The listing builds one solid part. Answer for the finished solid, in the listing's coordinates (mm). Round coordinates to 2 decimals unless told otherwise and drop trailing zeros. Loops run counter-clockwise (first coordinate to the right, second up) from the corner with the lowest first, then second, coordinate; pieces in that order, holes last. Notation, with made-up numbers: (-27, 35.25) -> (12, 35.25) arc R12 cw to (12, 44.25) -> close; hole circle Ø1 at (-6, 74). An arc over 180 degrees is marked (long way). Write each question's results on one line, items separated by ' | '. Start each with the question number.
(1) Straight lines are drawn through the part: probe 1 along X at (y, z) = (0.25, 183); probe 2 along Y at (x, z) = (-0.5, 208); probe 3 along Y at (x, z) = (-3.25, 251). For each, find the intervals that lie inside material, in ascending order.
(2) Flat-ended cylindrical pins translate along their axes: pin 1 (1.5 mm diameter, centred on y = -1.5, z = 77, fed in from +X); pin 2 (1.5 mm diameter, centred on y = 3.5, z = 240, fed in from +X); pin 3 (6 mm diameter, centred on x = 3.5, z = 210, fed in from +Y). Find the tip coordinate at first contact, or state that the pin passes through.
(3) The part is cut by section A-A (z = 55). Determine the outline of the cut face in (x, y).
```python
from build123d import *

# Parameters (mm, degrees)
CROQUIS1_R              = 5
SALIENTE_EXTRUIR1_DEPTH = 270


with BuildPart() as part:
    # Croquis1 → Saliente-Extruir1 (new body)
    with BuildSketch(Plane.XY):
        Circle(CROQUIS1_R)
    extrude(amount=SALIENTE_EXTRUIR1_DEPTH)

    # Cortar-Barrer1: sweep along a curve in space
    with BuildLine() as cortar_barrer1_path:
        ThreePointArc((5, 0, 270), (3.535533906, 3.535533906, 270), (0, 5, 270))
        ThreePointArc((0, 5, 270), (-3.535533906, 3.535533906, 270), (-5, 0, 270))
        ThreePointArc((-5, 0, 270), (-3.535533906, -3.535533906, 270), (0, -5, 270))
        ThreePointArc((0, -5, 270), (3.535533906, -3.535533906, 270), (5, 0, 270))
    # Croquis3 → Cortar-Barrer1 (sweep, cut)
    with BuildSketch(Plane(origin=(0, 0, 0), x_dir=(1, 0, 0), z_dir=(0, 1, 0))):
        Polygon((1.5, -270), (5, -267.999621553), (5, -270), align=None)
    sweep(path=cortar_barrer1_path.line, mode=Mode.SUBTRACT)

    # Cortar-Barrer2: sweep along a curve in space
    with BuildLine() as cortar_barrer2_path:
        ThreePointArc((5, 0, 0), (3.535533906, 3.535533906, 0), (0, 5, 0))
        ThreePointArc((0, 5, 0), (-3.535533906, 3.535533906, 0), (-5, 0, 0))
        ThreePointArc((-5, 0, 0), (-3.535533906, -3.535533906, 0), (0, -5, 0))
        ThreePointArc((0, -5, 0), (3.535533906, -3.535533906, 0), (5, 0, 0))
    # Croquis4 → Cortar-Barrer2 (sweep, cut)
    with BuildSketch(Plane(origin=(0, 0, 0), x_dir=(1, 0, 0), z_dir=(0, 1, 0))):
        Polygon((5, 0), (5, -2), (1.5, 0), align=None)
    sweep(path=cortar_barrer2_path.line, mode=Mode.SUBTRACT)


solid = part.part
```
Checked values:
1) probe 1: x = -4.99 to 4.99 | probe 2: y = -4.97 to 4.97 | probe 3: y = -3.8 to 3.8
2) pin 1: stops at x = 4.94 | pin 2: stops at x = 4.18 | pin 3: stops at y = 4.97
3) outline: circle Ø10 at (0, 0)
